Verification items for the finished model (mm, model axes). A direction names the side the tool comes from. Round coordinates to 2 decimals unless told otherwise and drop trailing zeros. Loops run counter-clockwise (first coordinate to the right, second up) from the corner with the lowest first, then second, coordinate; pieces in that order, holes last. Notation, with made-up numbers: M 40.25,27 L 69.25,27 A32 ccw 69.25,61 Z; hole C 31.25,10.5 d1. An arc over 180 degrees is marked long. Answer as CSV lines item,"result".
```python
from build123d import *

# Parameters (mm, degrees)
BOSS_EXTRUDE1_DEPTH = 4
SKETCH2_W           = 8.95
SKETCH2_H           = 19.3
SKETCH2_R           = 2.25
BOSS_EXTRUDE2_DEPTH = 4
FILLET1_R           = 10
FILLET2_R           = 4
SKETCH3_W           = 58.4
SKETCH3_H           = 19.3
SKETCH3_R           = 2
BOSS_EXTRUDE3_DEPTH = 4
CUT_EXTRUDE1_REACH  = 81.715
FILLET3_R           = 10


with BuildPart() as part:
    # Sketch1 → Boss-Extrude1 (new body)
    with BuildSketch(Plane(origin=(0, 0, 0), x_dir=(1, 0, 0), z_dir=(0, 1, 0))):
        Polygon((-49, 49.45), (-39, 49.45), (-39, 58.4), (0, 58.4), (0, 0), (-39, 0), (-39, 8.95), (-49, 8.95), align=None)
    extrude(amount=BOSS_EXTRUDE1_DEPTH)

    # Sketch2 → Boss-Extrude2 (add)
    # profile 1 of 2: a face of its own
    with BuildSketch(Plane.ZY.offset(39)):
        with Locations((-4.475, 13.65)):
            Rectangle(SKETCH2_W, SKETCH2_H)
        with Locations((-5, 18.55)):
            Circle(SKETCH2_R, mode=Mode.SUBTRACT)
        with Locations((-5, 8.55)):
            Circle(SKETCH2_R, mode=Mode.SUBTRACT)
    # profile 2 of 2: a face of its own
    with BuildSketch(Plane.ZY.offset(39)):
        with Locations((-53.925, 13.65)):
            Rectangle(SKETCH2_W, SKETCH2_H)
        with Locations((-54, 18.55)):
            Circle(SKETCH2_R, mode=Mode.SUBTRACT)
        with Locations((-54, 8.55)):
            Circle(SKETCH2_R, mode=Mode.SUBTRACT)
    extrude(amount=-BOSS_EXTRUDE2_DEPTH)

    # Fillet1
    # the kernel refuses this fillet: 10 mm, written as the material it adds along each edge
    with BuildSketch(Plane(origin=(-39, 0, -49.45), x_dir=(-1, 0, 0), z_dir=(0, 1, 0))) as fillet1_piece_1:
        with BuildLine():
            CenterArc((9.944722218, -10), FILLET1_R, 90, 83.97283344)
            Line((0, -8.95), (0, 0))
            Line((0, 0), (9.944722218, 0))
        make_face()
    extrude(amount=4)
    with BuildSketch(Plane(origin=(-39, 0, -8.95), x_dir=(0, 0, 1), z_dir=(0, 1, 0))) as fillet1_piece_2:
        with BuildLine():
            CenterArc((10, -9.944722218), FILLET1_R, 96.02716656, 83.97283344)
            Line((0, -9.944722218), (0, 0))
            Line((0, 0), (8.95, 0))
        make_face()
    extrude(amount=4)

    # Fillet2
    fillet2_edges = [part.edges().sort_by_distance(p)[0] for p in [
        (-37, 23.3, 0),
        (-37, 23.3, -58.4),
    ]]
    fillet(fillet2_edges, radius=FILLET2_R)

    # Sketch3 → Boss-Extrude3 (add)
    with BuildSketch(Plane(origin=(0, 0, 0), x_dir=(0, 0, -1), z_dir=(1, 0, 0))):
        with Locations((29.2, 13.65)):
            Rectangle(SKETCH3_W, SKETCH3_H)
        with Locations((39.95, 13.55)):
            Circle(SKETCH3_R, mode=Mode.SUBTRACT)
    extrude(amount=-BOSS_EXTRUDE3_DEPTH)

    # Sketch4 → Cut-Extrude1 (cut, up to next)
    with BuildSketch(Plane.XZ, mode=Mode.PRIVATE) as cut_extrude1_sk1:
        with BuildLine():
            Line((0, 0), (0, -20.5))
            Line((0, -20.5), (-23.45, -20.5))
            ThreePointArc((-23.45, -20.5), (-31.617083323, -17.117083323), (-35, -8.95))
            Line((-35, -8.95), (-35, 0))
            Line((-35, 0), (0, 0))
        make_face()
    cut_extrude1_tool1 = extrude(cut_extrude1_sk1.sketch, amount=-CUT_EXTRUDE1_REACH, mode=Mode.PRIVATE) & part.part
    add(cut_extrude1_tool1.solids().sort_by_distance((-16.879944, 0, -9.931243))[0], mode=Mode.SUBTRACT)

    # Fillet3
    fillet3_edges = [part.edges().sort_by_distance(p)[0] for p in [
        (-2, 23.3, -20.5),
        (-2, 23.3, -58.4),
    ]]
    fillet(fillet3_edges, radius=FILLET3_R)


solid = part.part
```
1) Section check B-B (y = 2.5). Record the cut outline in (x, z), plus the area to 3 significant figures.
Here are the results:
outline,"M -49,-49.45 L -48.94,-49.45 A10 cw -39,-58.4 L 0,-58.4 L 0,-20.5 L -23.45,-20.5 A11.55 cw -35,-8.95 L -35,0 L -39,0 A10 cw -48.94,-8.95 L -49,-8.95 Z"
area,"2,040 mm^2"
2) Section check D-D (x = -22.5). Record the cut outline in (y, z), plus the area to 3 significant figures.
Here are the results:
outline,"M 0,-58.4 L 4,-58.4 L 4,-20.5 L 0,-20.5 Z"
area,"152 mm^2"
3) Draft check along Y on faces 4 (the cylindrical face through (-37.028, 16.554, -3.962)), 5 (the flat face through (-37, 10, 0)), 6 (the flat face through (-2, 23.3, -39)). Enter one of: +Y half, -Y half, draft (parallel to the pull), parting line (faces both ways), or undercut.
Here are the results:
face 4,"undercut"
face 5,"draft"
face 6,"+Y half"
4) Section check A-A (z = -39.95). Record the cut outline in (x, y), plus the area to 3 significant figures.
Here are the results:
outline,"M -49,0 L 0,0 L 0,11.55 L -4,11.55 L -4,4 L -49,4 Z; M -4,15.55 L 0,15.55 L 0,23.3 L -4,23.3 Z"
area,"257 mm^2"
5) Section check C-C (y = 18.55). Record the cut outline in (x, z), plus the area to 3 significant figures.
Here are the results:
outline,"M -39,-58.4 L -35,-58.4 L -35,-56.25 L -39,-56.25 Z; M -39,-51.75 L -35,-51.75 L -35,-49.45 L -39,-49.45 Z; M -39,-8.95 L -35,-8.95 L -35,-7.25 L -39,-7.25 Z; M -39,-2.75 L -35,-2.75 L -35,0 L -39,0 Z; M -4,-56.91 L 0,-56.91 L 0,-21.99 L -4,-21.99 Z"
area,"175 mm^2"
6) Material ranges on probe 1 along Y at (x, z) = (-36, -54); probe 2 along Y at (x, z) = (-2.95, -39.95); probe 3 along X at (y, z) = (7.5, -26.5), recorded low to high.
Here are the results:
probe 1,"y = 0 to 6.3, 10.8 to 16.3, 20.8 to 23.3"
probe 2,"y = 0 to 11.55, 15.55 to 23.3"
probe 3,"x = -4 to 0"
7) Set-up check for faces 1 (the cylindrical face through (-37.028, 18.649, -56.248)), 2 (the flat face through (-35, 11, -5)), 3 (the flat face through (-39, 14, -5)): record each of +Z, -Z, +X, -X, +Y, -Y from which the full face is reachable in a straight line by a thin tool's end or side.
Here are the results:
face 1,"-X"
face 2,"+Z, +X, +Y, -Y"
face 3,"+Z, -Z, -X, +Y"
8) Go/stop test with flat-tipped pins: pin 1 (7 mm diameter, centred on y = 18.55, z = -54, fed in from -X); pin 2 (7 mm diameter, centred on y = 8.5, z = -6.5, fed in from +X); pin 3 (1.5 mm diameter, centred on x = -38, z = -35.5, fed in from +Y); pin 4 (3 mm diameter, centred on y = 12, z = -18, fed in from -X). Record where each tip stops, or that it passes through.
Here are the results:
pin 1,"stops at x = -39"
pin 2,"stops at x = -35"
pin 3,"stops at y = 4"
pin 4,"passes through"
